Answer from the drawing. Dimensions are ordinates in mm from the lowest x, y and z of the part. A direction names the side the tool comes from. Round coordinates to 2 decimals unless told otherwise and drop trailing zeros. Loops run counter-clockwise (first coordinate to the right, second up) from the corner with the lowest first, then second, coordinate; pieces in that order, holes last. Notation, with made-up numbers: M 85,7.25 L 111,7.25 A8 ccw 111,22.25 Z; hole C 31.25,11 d4. An arc over 180 degrees is marked long. Answer as CSV lines item,"result".
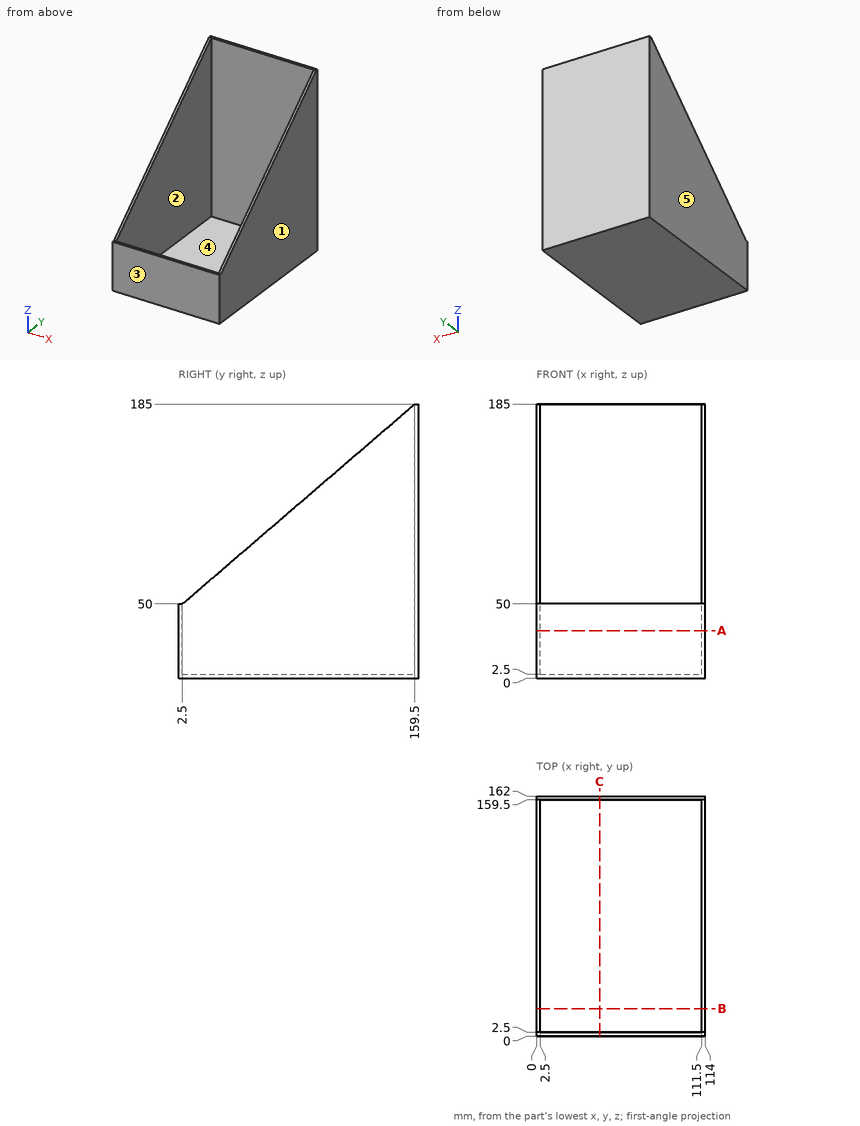
1) Find section A-A, the plane z = 32. Give the vertices of the cut face in (x, y), then the cut area to 4 significant figures.
Evaluation:
outline,"M 0,0 L 114,0 L 114,162 L 0,162 Z; hole M 2.5,2.5 L 111.5,2.5 L 111.5,159.5 L 2.5,159.5 Z"
area,"1,355 mm^2"
2) Find section B-B, the plane y = 18.5. Give the vertices of the cut face in (x, z), then the cut area to 3 significant figures.
Evaluation:
outline,"M 0,0 L 114,0 L 114,63.76 L 111.5,63.76 L 111.5,2.5 L 2.5,2.5 L 2.5,63.76 L 0,63.76 Z"
area,"591 mm^2"
3) Determine the mould class of the marked faces 3, 4 and 5 for opening direction X: released by +X, released by -X, zero draft, split by the parting line, or undercut.
Evaluation:
face 3,"zero draft"
face 4,"undercut"
face 5,"released by -X"
4) Find section C-C, the plane x = 42.5. Give the vertices of the cut face in (y, z).
Evaluation:
outline,"M 0,0 L 162,0 L 162,185 L 159.5,185 L 159.5,2.5 L 2.5,2.5 L 2.5,50 L 0,50 Z"
5) A tool of negligible diameter and unlimited length cuts with its end or side. For the marked faces 1 and 2, from which of +Z, -Z, +X, -X, +Y, -Y can it reach the whole face along a straight path? Write none if from no direction.
Evaluation:
face 1,"+Z, -Z, +X, +Y, -Y"
face 2,"+Z"
6) Straight lines are drawn through the part: line 1 (Y direction, x = 39, z = 27.5); line 2 (X direction, y = 140, z = 39); line 3 (Z direction, x = 99, y = 111.5). For each, find the intervals that lie inside material, in ascending order.
Evaluation:
line 1,"y = 0 to 2.5, 159.5 to 162"
line 2,"x = 0 to 2.5, 111.5 to 114"
line 3,"z = 0 to 2.5"
7) Each of these flat-tipped pins is pushed along its axis until it touches: P1, Ø10, axis at x = 93, z = 88.5, coming from the -Y side; P2, Ø1.2, axis at x = 63.5, y = 1, coming from the +Z side. Where does it stop, or does it pass through?
Evaluation:
P1,"stops at y = 159.5"
P2,"stops at z = 50"
